Verification items for this drawing (mm, ordinates from the low corner). Coordinates: 2 decimals unless noted, no trailing zeros. Write each loop counter-clockwise with the first axis right and the second up, starting at its lowest first coordinate (ties: lowest second). Pieces come first, ordered by that corner, then holes.
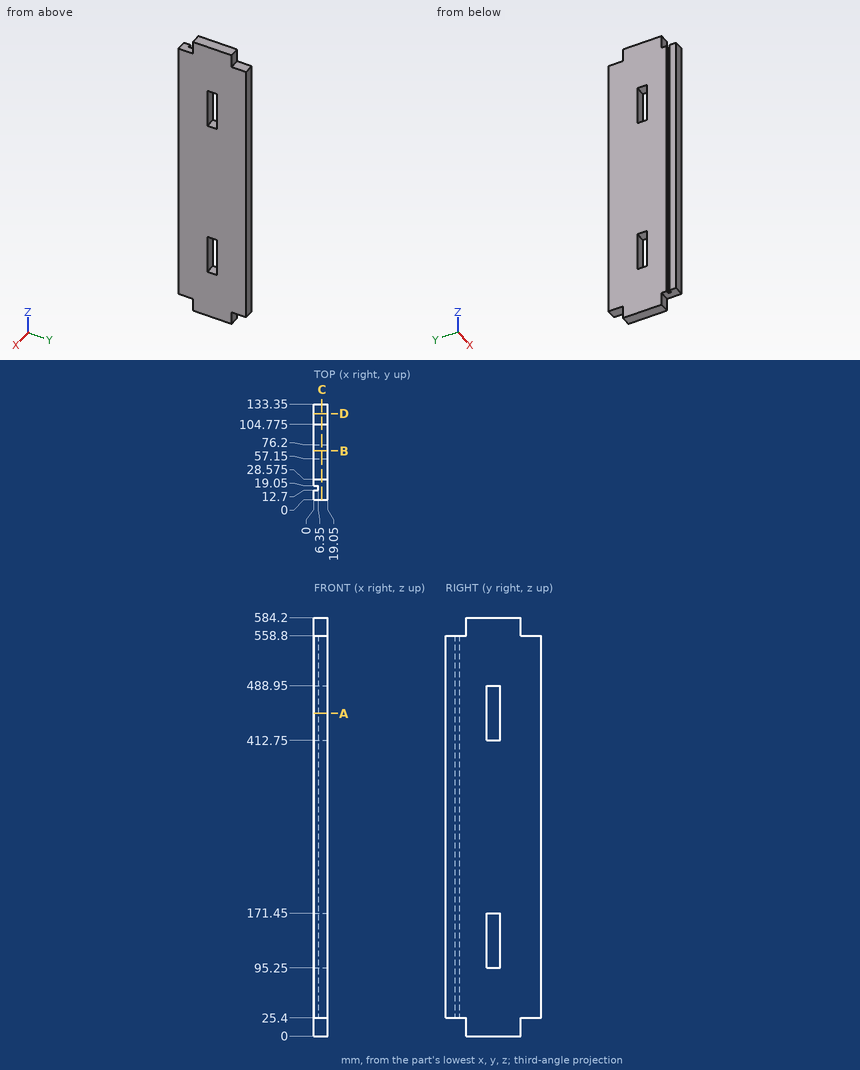
1. Gauge pin test, flat ends, axial feed: pin 1 Ø9.5 at (x, z) = (7.5, 16) entering from -Y (3 decimals); pin 2 Ø6 at (x, y) = (12.5, 21.5) entering from +Z; pin 3 Ø5.5 at (x, z) = (5, 576) entering from +Y (3 decimals); pin 4 Ø5.5 at (x, y) = (7.5, 66) entering from -Z. Record the tip position at first contact, or that the pin passes through.
Computed values:
pin 1: stops at y = 28.575
pin 2: stops at z = 558.8
pin 3: stops at y = 104.775
pin 4: stops at z = 0
2. Sectioned sample at C-C, the plane x = 11. Record the boundary of the cut face in (y, z) (3 decimals), and give its area (3 significant figures).
Computed values:
outline: (0, 25.4) - (28.575, 25.4) - (28.575, 0) - (104.775, 0) - (104.775, 25.4) - (133.35, 25.4) - (133.35, 558.8) - (104.775, 558.8) - (104.775, 584.2) - (28.575, 584.2) - (28.575, 558.8) - (0, 558.8) - close; hole (57.15, 95.25) - (76.2, 95.25) - (76.2, 171.45) - (57.15, 171.45) - close; hole (57.15, 412.75) - (76.2, 412.75) - (76.2, 488.95) - (57.15, 488.95) - close
area: 72,100 mm2
3. Sectioned sample at B-B, the plane y = 68. Record the boundary of the cut face in (x, z), and give its area (3 significant figures).
Computed values:
outline: (0, 0) - (19.05, 0) - (19.05, 95.25) - (0, 95.25) - close; (0, 171.45) - (19.05, 171.45) - (19.05, 412.75) - (0, 412.75) - close; (0, 488.95) - (19.05, 488.95) - (19.05, 584.2) - (0, 584.2) - close
area: 8,230 mm2
4. Sectioned sample at D-D, the plane y = 120. Record the boundary of the cut face in (x, z).
Computed values:
outline: (0, 25.4) - (19.05, 25.4) - (19.05, 558.8) - (0, 558.8) - close
5. Sectioned sample at A-A, the plane z = 450.5. Record the boundary of the cut face in (x, y).
Computed values:
outline: (0, 0) - (19.05, 0) - (19.05, 57.15) - (0, 57.15) - (0, 19.05) - (6.35, 19.05) - (6.35, 12.7) - (0, 12.7) - close; (0, 76.2) - (19.05, 76.2) - (19.05, 133.35) - (0, 133.35) - close
6. Thickness scan on line 1 along Z through (x, y) = (10.75, 64.5); line 2 along Y through (x, z) = (8.5, 475.5); line 3 along Y through (x, z) = (2.5, 446). Record the ranges inside material, lowest first.
Computed values:
line 1: z = 0 to 95.25, 171.45 to 412.75, 488.95 to 584.2
line 2: y = 0 to 57.15, 76.2 to 133.35
line 3: y = 0 to 12.7, 19.05 to 57.15, 76.2 to 133.35
